Autodesk Inventor part; units mm, degrees
ref_plane "YZ Plane" through (0, 0, 0) normal (1, 0, 0) x (0, 1, 0)
ref_plane "XZ Plane" through (0, 0, 0) normal (0, 1, 0) x (-1, 0, 0)
ref_plane "XY Plane" through (0, 0, 0) normal (0, 0, 1) x (1, 0, 0)
sketch "Esquisse1" plane through (0, 0, 0) normal (0, 1, 0) x (-1, 0, 0)
  line L0 (0, 0) -> (27, 0)
  line L1 (27, 0) -> (27, 66.5)
  line L2 (27, 66.5) -> (0, 66.5)
  line L3 (0, 66.5) -> (0, 0)
  line L4 (4.65, 63.35) -> (22.35, 63.35) construction
  line L5 (22.35, 63.35) -> (22.35, 3.15) construction
  line L6 (22.35, 3.15) -> (4.65, 3.15) construction
  line L7 (4.65, 3.15) -> (4.65, 63.35) construction
  line L8 (13.5, 63.35) -> (13.5, 66.5) construction
  line L9 (22.35, 33.25) -> (27, 33.25) construction
  line L10 (4.65, 33.25) -> (0, 33.25) construction
  line L11 (13.5, 3.15) -> (13.5, 0) construction
  circle A0 centre (4.65, 63.35) radius 2.15
  circle A1 centre (22.35, 63.35) radius 2.15
  circle A2 centre (4.65, 3.15) radius 2.15
  circle A3 centre (22.35, 3.15) radius 2.15
  dimension "d0" = 27
  dimension "d1" = 66.5
  dimension "d2" = 60.2
  dimension "d3" = 17.7
  dimension "d4" = 4.3
extrude "Extrusion1" add sketch "Esquisse1" along normal blind 1.6
fillet "Congé1" radius 2 4 edges at (0, 0.8, 0) (-27, 0.8, 0) (0, 0.8, 66.5) (-27, 0.8, 66.5)
sketch "Esquisse2" plane through (0, 1.6, 0) normal (0, 1, 0) x (1, 0, 0)
  line L0 (-2, 0) -> (-25, 0) construction
  line L1 (-18.5, 0) -> (-8.5, 0)
  line L2 (-8.5, 0) -> (-8.5, -5)
  line L3 (-8.5, -5) -> (-18.5, -5)
  line L4 (-18.5, -5) -> (-18.5, 0)
  point P0 (0, 0)
  point P1 (-13.5, 0)
  dimension "d8" = 5
  dimension "d9" = 10
extrude "Extrusion2" add sketch "Esquisse2" along normal blind 2
sketch "Esquisse3" plane through (0, 1.6, 0) normal (0, 1, 0) x (1, 0, 0)
  line L0 (-6.6018, -5.2) -> (-6.6018, -9.2)
  line L1 (-6.6018, -9.2) -> (-20.6018, -9.2)
  line L2 (-20.6018, -9.2) -> (-20.6018, -5.2)
  line L3 (-18.5, -5) -> (-8.5, -5)
  line L4 (-17.7303, -5) -> (-13.5194, -5) construction
  line L5 (-13.6018, -9.2) -> (-13.6018, -29.6083) construction
  line L6 (-19.6018, -9.2) -> (-23.6018, -9.2)
  line L7 (-23.6018, -9.2) -> (-23.6018, -29.2)
  line L8 (-23.6018, -29.2) -> (-19.6018, -29.2)
  line L9 (-19.6018, -29.2) -> (-19.6018, -9.2)
  line L10 (-7.6018, -9.2) -> (-3.6018, -9.2)
  line L11 (-3.6018, -9.2) -> (-3.6018, -29.2)
  line L12 (-3.6018, -29.2) -> (-7.6018, -29.2)
  line L13 (-7.6018, -29.2) -> (-7.6018, -9.2)
  line L14 (-8.5, -5) -> (-18.5, -5)
  line L15 (-20.6018, -5.2) -> (-6.6018, -5.2)
  point P0 (0, 0)
  point P1 (-13.5, -5)
  dimension "d12" = 14
  dimension "d13" = 4
  dimension "d14" = 20
  dimension "d15" = 4
  dimension "d16" = 12
  dimension "d19" = 0.2
extrude "Extrusion3" add sketch "Esquisse3" along normal blind 2
properties part number "opencm"
The listing builds one solid part. Answer for the finished solid, in the listing's coordinates (mm). A direction names the side the tool comes from. Round coordinates to 2 decimals unless told otherwise and drop trailing zeros. Order: outer loops, then holes, each group sorted by start corner. A loop starts at its lowest first (then second) coordinate and runs counter-clockwise, first axis right, second up. Notation, with made-up numbers: (-33, -12.5) -> (-5, -12.5) arc R26 cw to (-5, 5.5) -> close; hole circle Ø6 at (89.5, 33). An arc over 180 degrees is marked (long way). Write each question's results on one line, items separated by ' | '. Start each with the question number.
Q1. Find section C-C (x = -4.65). Determine the outline of the cut face in (y, z).
Q2. Find section D-D (x = -16.75). Determine the outline of the cut face in (y, z).
Q3. Find section B-B (y = 2.45). Determine the outline of the cut face in (x, z), then the cut area to 3 significant figures.
Q4. Straight lines are drawn through the part: probe 1 along Z at (x, y) = (-4.65, 0.6); probe 2 along X at (y, z) = (3.4, 27); probe 3 along Z at (x, y) = (-13, 1.65). For each, find the intervals that lie inside material, in ascending order. Write a range as from..to.
Q5. Which of the six approach directions +Z, -Z, +X, -X, +Y, -Y give full straight-line access (tool end or side, diameter ignored) to faces 1 (the flat face through (-8.5, 3, 2)), 2 (the flat face through (-20.602, 3, 7)), 3 (the flat face through (-7.602, 3, 19)), 4 (the flat face through (-3.602, 3, 19)), 5 (the flat face through (-13, 3, 5))?
Q6. Find section A-A (z = 3.15). Determine the outline of the cut face in (x, y).
Q7. The mould has two halves that part along X. Classify faces 6 (the flat face through (-13, 1.6, 34)), 7 (the flat face through (-23.602, 3, 19)), 8 (the flat face through (-6, 3, 29.2)): pulls with the +X half, pulls with the -X half, needs draft (parallel to the pull), parting line crosses it, or undercut.
Q8. Each of these flat-tipped pins is pushed along its axis until it touches: pin 1 (1 mm diameter, centred on x = -6.5, y = 2.5, fed in from +Z); pin 2 (0.6 mm diameter, centred on y = 3, z = 20, fed in from -X); pin 3 (1.6 mm diameter, centred on y = 2.5, z = 24, fed in from +X). Where does it stop, or does it pass through?
Worked answers:
1) outline: (0, 0) -> (1.6, 0) -> (1.6, 1) -> (0, 1) -> close; (0, 5.3) -> (1.6, 5.3) -> (1.6, 9.2) -> (3.6, 9.2) -> (3.6, 29.2) -> (1.6, 29.2) -> (1.6, 61.2) -> (0, 61.2) -> close; (0, 65.5) -> (1.6, 65.5) -> (1.6, 66.5) -> (0, 66.5) -> close
2) outline: (0, 0) -> (3.6, 0) -> (3.6, 5) -> (1.6, 5) -> (1.6, 5.2) -> (3.6, 5.2) -> (3.6, 9.2) -> (1.6, 9.2) -> (1.6, 66.5) -> (0, 66.5) -> close
3) outline: (-23.6, 9.2) -> (-20.6, 9.2) -> (-20.6, 5.2) -> (-6.6, 5.2) -> (-6.6, 9.2) -> (-3.6, 9.2) -> (-3.6, 29.2) -> (-7.6, 29.2) -> (-7.6, 9.2) -> (-19.6, 9.2) -> (-19.6, 29.2) -> (-23.6, 29.2) -> close; (-18.5, 0) -> (-8.5, 0) -> (-8.5, 5) -> (-18.5, 5) -> close | area: 266 mm2
4) probe 1: z = 0..1, 5.3..61.2, 65.5..66.5 | probe 2: x = -23.6..-19.6, -7.6..-3.6 | probe 3: z = 0..5, 5.2..9.2
5) face 1: -Z, +X, +Y | face 2: -Z, -X, +Y | face 3: +Z, +Y | face 4: +Z, -Z, +X, +Y | face 5: +X, -X, +Y
6) outline: (-27, 0) -> (-24.5, 0) -> (-24.5, 1.6) -> (-27, 1.6) -> close; (-20.2, 0) -> (-6.8, 0) -> (-6.8, 1.6) -> (-8.5, 1.6) -> (-8.5, 3.6) -> (-18.5, 3.6) -> (-18.5, 1.6) -> (-20.2, 1.6) -> close; (-2.5, 0) -> (0, 0) -> (0, 1.6) -> (-2.5, 1.6) -> close
7) face 6: undercut | face 7: pulls with the -X half | face 8: needs draft
8) pin 1: stops at z = 29.2 | pin 2: stops at x = -23.6 | pin 3: stops at x = -3.6
